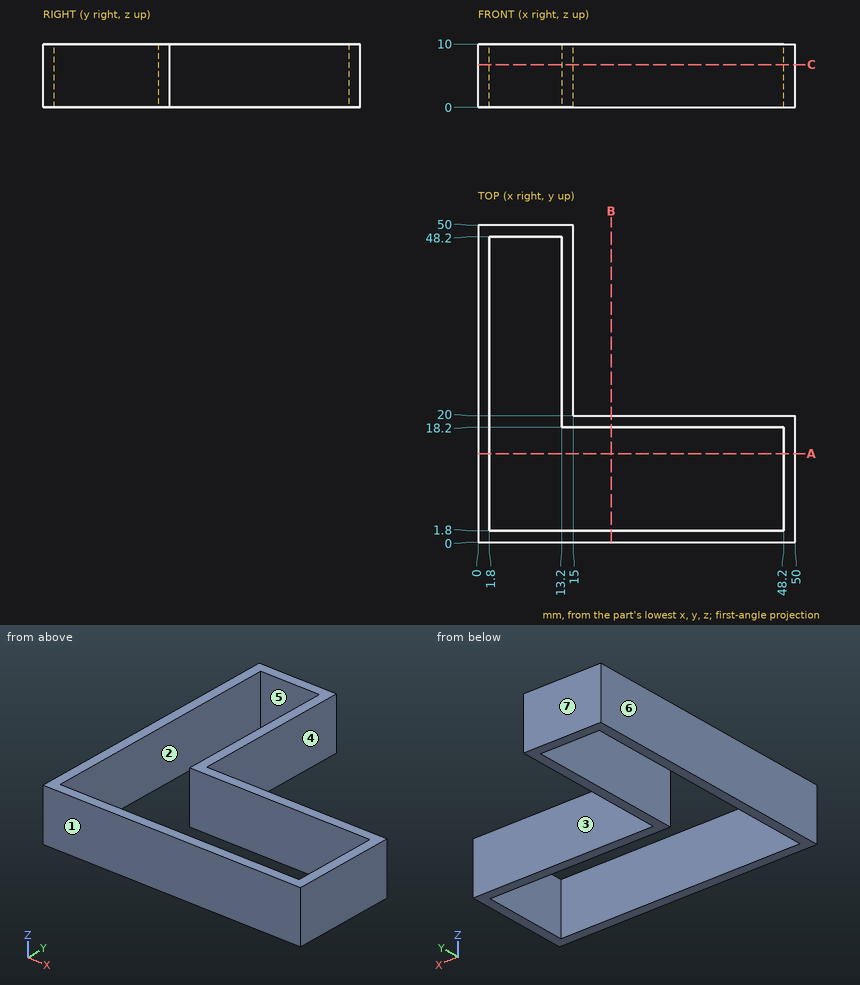
Check sheet for the drawn part. Datum: minimum x, y, z corner. Units: mm. A direction names the side the tool comes from. Round coordinates to 2 decimals unless told otherwise and drop trailing zeros. Write each loop counter-clockwise with the first axis right and the second up, starting at its lowest first coordinate (ties: lowest second). Pieces come first, ordered by that corner, then holes. Notation, with made-up numbers: (-9.5, 84) -> (43.5, 84) arc R22 cw to (43.5, 107) -> close; hole circle Ø2 at (13.5, 70). An arc over 180 degrees is marked (long way). One line per item, written item: value. Start each with the question number.
(1) Scan lines: line 1 (Y direction, x = 27, z = 3.75); line 2 (X direction, y = 11, z = 3.5); line 3 (X direction, y = 44, z = 5). Record each from-to range of solid material in increasing order. Write a range as [from, to].
(2) Cross-section at B-B, the plane x = 21. Record the cut outline in (y, z), and give its area (3 significant figures).
(3) Cross-section at C-C, the plane z = 6.75. Record the cut outline in (x, y), and give its area (3 significant figures).
(4) Cross-section at A-A, the plane y = 14. Record the cut outline in (x, z).
(5) Draft check along X on the marked faces 4, 5, 6 and 7. Enter one of: +X half, -X half, draft (parallel to the pull), parting line (faces both ways), or undercut.
(6) Access from +Z, -Z, +X, -X, +Y, -Y to the whole of each face (thin tool, end or side, straight path). Record for the marked faces 1, 2 and 3.
(7) Go/stop test with flat-tipped pins: pin 1 Ø2 at (y, z) = (36.5, 4) entering from -X; pin 2 Ø3 at (y, z) = (23.5, 7) entering from +X; pin 3 Ø6 at (x, z) = (21, 1.5) entering from +Y. Record where each tip stops, or that it passes through.
Answer:
1. line 1: [0, 1.8], [18.2, 20]
1. line 2: [0, 1.8], [48.2, 50]
1. line 3: [0, 1.8], [13.2, 15]
2. outline: (0, 0) -> (1.8, 0) -> (1.8, 10) -> (0, 10) -> close; (18.2, 0) -> (20, 0) -> (20, 10) -> (18.2, 10) -> close
2. area: 36.0 mm²
3. outline: (0, 0) -> (50, 0) -> (50, 20) -> (15, 20) -> (15, 50) -> (0, 50) -> close; hole (1.8, 1.8) -> (48.2, 1.8) -> (48.2, 18.2) -> (13.2, 18.2) -> (13.2, 48.2) -> (1.8, 48.2) -> close
3. area: 347 mm²
4. outline: (0, 0) -> (1.8, 0) -> (1.8, 10) -> (0, 10) -> close; (48.2, 0) -> (50, 0) -> (50, 10) -> (48.2, 10) -> close
5. face 4: +X half
5. face 5: undercut
5. face 6: -X half
5. face 7: draft
6. face 1: +Z, -Z, +X, -X, -Y
6. face 2: +Z, -Z
6. face 3: +Z, -Z, +X, +Y
7. pin 1: x = 0
7. pin 2: x = 15
7. pin 3: y = 20
